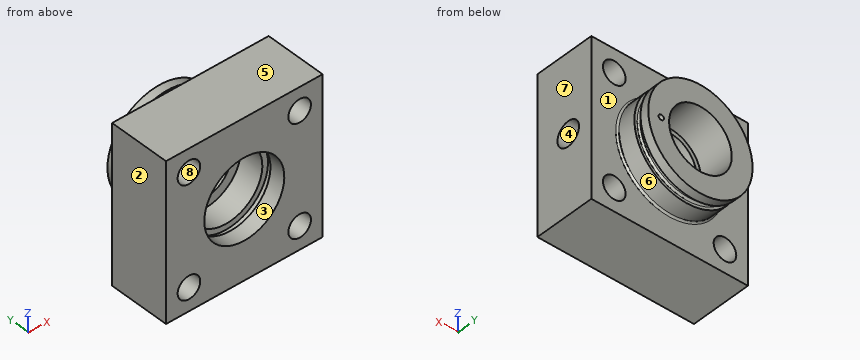
from build123d import *

# Parameters (mm, degrees)
SKETCH1_W                  = 90
SKETCH1_H                  = 90
EXTRUDE1_DEPTH             = 35
SKETCH2_R                  = 30
EXTRUDE2_DEPTH             = 20
SKETCH5_W                  = 6.681632653
SKETCH5_H                  = 4
SKETCH6_R                  = 6.5
CUT_EXTRUDE1_DEPTH         = 85.113019206
MIRROR2_COPY_1_SKETCH_R    = 6.5
MIRROR2_COPY_1_DEPTH       = 85.113019206
M16X2_0_TAPPED_HOLE1_D     = 14
M16X2_0_TAPPED_HOLE1_DEPTH = 18
M16X2_0_TAPPED_HOLE1_TIP   = 4.206024333
FILLET1_R                  = 1
CUT_SWEEP1_START           = -49.987863257
CUT_SWEEP1_OUTLINE_R       = 1.5
CUT_SWEEP1_DEPTH           = 29.274008659


# Read off the part's stored shape, not the designer's step: Cut-Sweep1
with BuildPart() as part:
    # Sketch1 → Extrude1 (new body)
    with BuildSketch(Plane(origin=(0, 0, 0), x_dir=(1, 0, 0), z_dir=(0, 1, 0))):
        Rectangle(SKETCH1_W, SKETCH1_H)
    extrude(amount=EXTRUDE1_DEPTH)

    # Sketch2 → Extrude2 (add)
    with BuildSketch(Plane(origin=(0, 35, 0), x_dir=(-1, 0, 0), z_dir=(0, 1, 0))):
        with Locations(Location((0, 0, 0), (0, 0, 270))):
            Circle(SKETCH2_R)
    extrude(amount=EXTRUDE2_DEPTH)

    # Sketch3 → Cut-Revolve1 (revolve, cut)
    with BuildSketch(Plane.XY, mode=Mode.PRIVATE) as cut_revolve1_sk:
        Polygon((0, 0), (-23, 0), (-23, 9), (-24.25, 9), (-24.25, 12), (-21, 12), (-21, 26), (-15.5, 26), (-15.5, 35), (-18, 35), (-18, 55), (0, 55), align=None)
    revolve(cut_revolve1_sk.sketch.rotate(Axis((0, 0, 0), (0, 1, 0)), 270), axis=Axis((0, 0, 0), (0, 1, 0)), mode=Mode.SUBTRACT)

    # Sketch5 → Cut-Revolve2 (revolve, cut)
    with BuildSketch(Plane.XY, mode=Mode.PRIVATE) as cut_revolve2_sk:
        with Locations((-30.740816327, 48)):
            Rectangle(SKETCH5_W, SKETCH5_H)
    revolve(cut_revolve2_sk.sketch.rotate(Axis((0, 0, 0), (0, 1, 0)), 270), axis=Axis((0, 0, 0), (0, 1, 0)), mode=Mode.SUBTRACT)

    # Sketch6 → Cut-Extrude1 (cut, through all)
    with BuildSketch(Plane.XZ):
        with Locations(Location((31.819805153, -31.819805153, 0), (0, 0, 270))):
            Circle(SKETCH6_R)
    cut_extrude1 = extrude(amount=-CUT_EXTRUDE1_DEPTH, mode=Mode.SUBTRACT)

    # Mirror1: Cut-Extrude1 across plane
    add(cut_extrude1.mirror(Plane.XY), mode=Mode.SUBTRACT)

    # Mirror2: Cut-Extrude1 across plane
    add(cut_extrude1.mirror(Plane(origin=(0, 0, 0), x_dir=(0, 0, 1), z_dir=(1, 0, 0))), mode=Mode.SUBTRACT)

    # Mirror2 copy 1 sketch → Mirror2 copy 1 (cut, through all)
    with BuildSketch(Plane(origin=(0, 0, 0), x_dir=(-1, 0, 0), z_dir=(0, -1, 0))):
        with Locations(Location((31.819805153, -31.819805153, 0), (0, 0, 270))):
            Circle(MIRROR2_COPY_1_SKETCH_R)
    extrude(amount=-MIRROR2_COPY_1_DEPTH, mode=Mode.SUBTRACT)

    # M16x2.0 Tapped Hole1
    with Locations(Plane(origin=(45, 0, 0), x_dir=(0, 0, -1), z_dir=(1, 0, 0))):
        with Locations((0, 20)):
            Hole(M16X2_0_TAPPED_HOLE1_D / 2, depth=M16X2_0_TAPPED_HOLE1_DEPTH)
            with Locations((0, 0, -(M16X2_0_TAPPED_HOLE1_DEPTH + M16X2_0_TAPPED_HOLE1_TIP / 2))):  # 118° drill point
                Cone(0, M16X2_0_TAPPED_HOLE1_D / 2, M16X2_0_TAPPED_HOLE1_TIP, mode=Mode.SUBTRACT)

    # Fillet1
    fillet1_edges = [part.edges().sort_by_distance(p)[0] for p in [
        (0, 35, 30),
        (0, 50, 27.4),
        (0, 46, 27.4),
    ]]
    fillet(fillet1_edges, radius=FILLET1_R)

    # Cut-Sweep1 outline → Cut-Sweep1 (cut)
    with BuildSketch(Plane(origin=(0, 0, 0), x_dir=(0.981627183447665, 0.19080899537653903, 0), z_dir=(0.19080899537653903, -0.9816271834476651, 0)).offset(CUT_SWEEP1_START)):
        with Locations((32.581106373, 0)):
            Circle(CUT_SWEEP1_OUTLINE_R)
    extrude(amount=CUT_SWEEP1_DEPTH, mode=Mode.SUBTRACT)


solid = part.part
Model file for the job. Use its own axes, mm. Face numbers are marked on the shaded views. A direction names the side the tool comes from. Coordinates: 2 decimals unless noted, no trailing zeros. Write each loop counter-clockwise with the first axis right and the second up, starting at its lowest first coordinate (ties: lowest second). Pieces come first, ordered by that corner, then holes. Notation, with made-up numbers: (-35, -16.5) -> (-25, -16.5) arc R5 ccw to (-25, -12.5) -> close; hole circle Ø7 at (-26, 48.5). An arc over 180 degrees is marked (long way). One line per item, written item: value. Start each with the question number.
1) Which spindle directions (+Z, -Z, +X, -X, +Y, -Y) get a long thin tool onto all of the face, cutting with end or side? Do the marked faces 1, 2, 3 and 4. Say none if no direction does.
2) Flat gauge pins, fed straight in: pin 1 Ø2 at (x, z) = (23.5, 12) entering from -Y; pin 2 Ø6 at (x, z) = (-34, 7) entering from +Y; pin 3 Ø25 at (x, z) = (0, 0) entering from -Y; pin 4 Ø1.5 at (x, z) = (18.5, 3.5) entering from -Y. Where does each tip first touch, or does it go through?
3) Pull direction Z, two halves, no side cores. Call the marked faces 5, 6, 7 and 8: +Z half, -Z half, draft (parallel to the pull), parting line (faces both ways), or undercut.
4) Probe probe 1 along X at (y, z) = (22, -28.5); probe 2 along Y at (x, z) = (-22, -7); probe 3 along Z at (x, y) = (-35.5, 22.5). List the from-to ranges inside material, lowest first.
5) Slice it at A-A on x = 35.5. Write the cut outline in (y, z), then the cut area to 3 significant figures.
6) Slice it at B-B on z = -35. Write the cut outline in (x, y), then the cut area to 3 significant figures.
Answers follow:
1. face 1: +Y
1. face 2: +Z, -Z, -X, +Y, -Y
1. face 3: -Y
1. face 4: +X
2. pin 1: y = 0
2. pin 2: y = 35
2. pin 3: through
2. pin 4: y = 26
3. face 5: +Z half
3. face 6: parting line
3. face 7: draft
3. face 8: undercut
4. probe 1: -45 to -37.41, -26.23 to 26.23, 37.41 to 45
4. probe 2: 0 to 9, 12 to 55
4. probe 3: -45 to -37.18, -26.46 to 26.46, 37.18 to 45
5. outline: (0, -45) -> (35, -45) -> (35, -37.18) -> (0, -37.18) -> close; (0, -26.46) -> (35, -26.46) -> (35, 26.46) -> (0, 26.46) -> close; (0, 37.18) -> (35, 37.18) -> (35, 45) -> (0, 45) -> close; hole circle Ø14 at (20, 0)
5. area: 2,250 mm2
6. outline: (-45, 0) -> (-37.49, 0) -> (-37.49, 35) -> (-45, 35) -> close; (-26.15, 0) -> (26.15, 0) -> (26.15, 35) -> (-26.15, 35) -> close; (37.49, 0) -> (45, 0) -> (45, 35) -> (37.49, 35) -> close
6. area: 2,360 mm2
